Work out the finished part from the listing and answer in its coordinate system (mm). A direction names the side the tool comes from. Coordinates: 2 decimals unless noted, no trailing zeros. Write each loop counter-clockwise with the first axis right and the second up, starting at its lowest first coordinate (ties: lowest second). Pieces come first, ordered by that corner, then holes. Notation, with made-up numbers: (-30.75, -34.75) - (-25.75, -34.75) arc R11 cw to (-25.75, -30.75) - close; hole circle Ø9 at (8.5, -27.75). An arc over 180 degrees is marked (long way). Use one line per item in the form item = value. Start each with the question number.
Item 1: Determine the mould class of faces 4 (the flat face through (-1, -20, 4)), 5 (the cylindrical face through (-43.298, 0.101, 22.075)), 6 (the flat face through (-55, 0, 4)), 7 (the cylindrical face through (4.504, 0.189, 21.117)) for opening direction X: released by +X, released by -X, zero draft, split by the parting line, or undercut.
Item 2: A cutting plane is placed at B-B (x = -23.55). Write down the section's boundary in (y, z).
Item 3: A cutting plane is placed at D-D (x = 8.8). Write down the section's boundary in (y, z).
Item 4: A cutting plane is placed at C-C (y = -9). Write down the section's boundary in (x, z), then the cut area to 3 significant figures.
Item 5: Given pin 1 (8 mm diameter, centred on x = 37, y = 12.5, fed in from +Z); pin 2 (2.5 mm diameter, centred on x = -15.5, y = 0.5, fed in from +Z); pin 3 (13.5 mm diameter, centred on x = 40, y = -3.5, fed in from +Z); pin 4 (2 mm diameter, centred on x = -23.55, y = 0, fed in from -Z), each flat-ended and moving along its own axis, determine where each tip first touches the part or whether it passes through.
Item 6: Consider probe 1 along Y at (x, z) = (-41, 21.5); probe 2 along X at (y, z) = (0, 3); probe 3 along X at (y, z) = (0, 2). Determine where each line is inside the solid, lowest interval first.
Item 7: A cutting plane is placed at A-A (z = 30). Write down the section's boundary in (x, y).
Item 8: For faces 1 (the cylindrical face through (50.217, -0.67, 7.51)), 2 (the flat face through (34, 0, 9.4)), 3 (the flat face through (26, 0, 5.2)), determine the directions among +Z, -Z, +X, -X, +Y, -Y from which every point of the face is accessible in a straight line to the end or side of a thin tool.
from build123d import *

# Parameters (mm, degrees)
F0_W      = 110
F0_H      = 40
F1_DEPTH  = 8.2
F2_R      = 6
F3_R      = 4.3
F4_DEPTH  = 26.2
F5_R      = 2.55
F5_R_2    = 4
F6_DEPTH  = 6.8
F7_R      = 1.75
F8_DEPTH  = 8.201
F10_DEPTH = 40.001
F11_R     = 2.3
F12_DEPTH = 25


with BuildPart() as f1:
    # F0 (on Top) → F1 (new body)
    with BuildSketch(Plane.XY):
        Rectangle(F0_W, F0_H)
    extrude(amount=F1_DEPTH)

    # F2
    f2_edges = [f1.edges().sort_by_distance(p)[0] for p in [
        (55, 0, 0),
    ]]
    fillet(f2_edges, radius=F2_R)

    # F3 (on face) → F4 (join)
    with BuildSketch(Plane.XY.offset(8.2)):
        with Locations((-41, 0)):
            Circle(F3_R)
        with Locations((-16.1, 0)):
            Circle(F3_R)
        with Locations((8.8, 0)):
            Circle(F3_R)
        with Locations((33.7, 0)):
            Circle(F3_R)
    extrude(amount=F4_DEPTH)

    # F5 (on face) → F6 (cut)
    with BuildSketch(Plane(origin=(0, 0, 0), x_dir=(1, 0, 0), z_dir=(0, 0, -1))):
        with Locations((48.6, 0)):
            Circle(F5_R)
        with Locations((21.05, 0)):
            Circle(F5_R_2)
        with Locations((-23.55, 0)):
            Circle(F5_R_2)
    extrude(amount=-F6_DEPTH, mode=Mode.SUBTRACT)

    # F7 (on face) → F8 (cut, through all)
    with BuildSketch(Plane.XY.offset(8.2)):
        with Locations((48.6, 0)):
            Circle(F7_R)
        with Locations((21.05, 0)):
            Circle(F7_R)
        with Locations((-23.55, 0)):
            Circle(F7_R)
    extrude(amount=-F8_DEPTH, mode=Mode.SUBTRACT)

    # F9 (on face) → F10 (cut, through all)
    with BuildSketch(Plane.XZ.offset(20)):
        Polygon((-32.3, 8.2), (-36.3, 8.2), (-35.5, 5.2), (-33.1, 5.2), align=None)
        Polygon((27.9, 8.2), (23.9, 8.2), (24.7, 5.2), (27.1, 5.2), align=None)
    extrude(amount=-F10_DEPTH, mode=Mode.SUBTRACT)

    # F11 (on face) → F12 (cut)
    with BuildSketch(Plane.XY.offset(34.4)):
        with Locations((-41, 0)):
            Circle(F11_R)
        with Locations((-16.1, 0)):
            Circle(F11_R)
        with Locations((8.8, 0)):
            Circle(F11_R)
        with Locations((33.7, 0)):
            Circle(F11_R)
    extrude(amount=-F12_DEPTH, mode=Mode.SUBTRACT)


solid = f1.part
Answer:
q1.face_4 = zero draft
q1.face_5 = undercut
q1.face_6 = released by -X
q1.face_7 = undercut
q2.outline = (-20, 0) - (-4, 0) - (-4, 6.8) - (-1.75, 6.8) - (-1.75, 8.2) - (-20, 8.2) - close; (1.75, 6.8) - (4, 6.8) - (4, 0) - (20, 0) - (20, 8.2) - (1.75, 8.2) - close
q3.outline = (-20, 0) - (20, 0) - (20, 8.2) - (4.3, 8.2) - (4.3, 34.4) - (2.3, 34.4) - (2.3, 9.4) - (-2.3, 9.4) - (-2.3, 34.4) - (-4.3, 34.4) - (-4.3, 8.2) - (-20, 8.2) - close
q4.outline = (-55, 0) - (49, 0) arc R6 ccw to (55, 6) - (55, 8.2) - (27.9, 8.2) - (27.1, 5.2) - (24.7, 5.2) - (23.9, 8.2) - (-32.3, 8.2) - (-33.1, 5.2) - (-35.5, 5.2) - (-36.3, 8.2) - (-55, 8.2) - close
q4.area = 875 mm²
q5.pin_1 = 8.2
q5.pin_2 = 9.4
q5.pin_3 = 34.4
q5.pin_4 = through
q6.probe_1 = -4.3 to -2.3, 2.3 to 4.3
q6.probe_2 = -55 to -27.55, -19.55 to 17.05, 25.05 to 46.05, 51.15 to 54.2
q6.probe_3 = -55 to -27.55, -19.55 to 17.05, 25.05 to 46.05, 51.15 to 53.47
q7.outline = circle Ø8.6 at (-41, 0); circle Ø8.6 at (-16.1, 0); circle Ø8.6 at (8.8, 0); circle Ø8.6 at (33.7, 0); hole circle Ø4.6 at (-41, 0); hole circle Ø4.6 at (-16.1, 0); hole circle Ø4.6 at (8.8, 0); hole circle Ø4.6 at (33.7, 0)
q8.face_1 = +Z, -Z
q8.face_2 = +Z
q8.face_3 = +Z, +Y, -Y
